Could you check a few things on this model? Use its own coordinates, in mm. A direction names the side the tool comes from. Coordinates: 2 decimals unless noted, no trailing zeros. Loops run counter-clockwise (first coordinate to the right, second up) from the corner with the lowest first, then second, coordinate; pieces in that order, holes last. Notation, with made-up numbers: (89, 54.25) -> (134, 54.25) arc R23 cw to (134, 86.25) -> close; hole circle Ø5 at (-25, 63). An arc over 180 degrees is marked (long way). One line per question, with ' | ' between items.
```python
from build123d import *

# Parameters (mm, degrees)
SKETCH1_R           = 8
BOSS_EXTRUDE1_DEPTH = 67
SKETCH2_R           = 3
BOSS_EXTRUDE2_DEPTH = 2.5
SKETCH3_R           = 3
BOSS_EXTRUDE3_DEPTH = 2.5
SKETCH4_R           = 2
BOSS_EXTRUDE4_DEPTH = 13


with BuildPart() as part:
    # Sketch1 → Boss-Extrude1 (new body)
    with BuildSketch(Plane.XY):
        Circle(SKETCH1_R)
    extrude(amount=BOSS_EXTRUDE1_DEPTH)

    # Sketch2 → Boss-Extrude2 (add)
    with BuildSketch(Plane.XY.offset(67)):
        Circle(SKETCH2_R)
    extrude(amount=BOSS_EXTRUDE2_DEPTH)

    # Sketch3 → Boss-Extrude3 (add)
    with BuildSketch(Plane(origin=(0, 0, 0), x_dir=(-1, 0, 0), z_dir=(0, 0, -1))):
        Circle(SKETCH3_R)
    extrude(amount=BOSS_EXTRUDE3_DEPTH)

    # Sketch4 → Boss-Extrude4 (add)
    with BuildSketch(Plane(origin=(0, 0, -2.5), x_dir=(-1, 0, 0), z_dir=(0, 0, -1))):
        Circle(SKETCH4_R)
    extrude(amount=BOSS_EXTRUDE4_DEPTH)


solid = part.part
```
Q1. Imagine slicing it at D-D on z = -4.5. Write out the boundary of the cut face in (x, y), plus the area to 3 significant figures.
Values follow:
outline: circle Ø4 at (0, 0) | area: 12.6 mm2
Q2. Please list where these lines run through material, in increasing order: L1, parallel to Z at x = 1.5, y = -6.5; L2, parallel to Y at x = -7, z = 1; L3, parallel to Y at x = -5.25, z = 28. Write a range as [from, to].
Values follow:
L1: z = [0, 67] | L2: y = [-3.87, 3.87] | L3: y = [-6.04, 6.04]
Q3. For faces 1 (the face through (0, 0, 69.5)), 2 (the face through (0, -2, -9)), 3 (the face through (3.4, 0.1, 67)), which set-ups out of +Z, -Z, +X, -X, +Y, -Y let a thin tool reach every point of the face, with its end or its side?
Values follow:
face 1: +Z, +X, -X, +Y, -Y | face 2: -Z | face 3: +Z
Q4. Imagine slicing it at C-C on z = 51.5. Write out the boundary of the cut face in (x, y).
Values follow:
outline: circle Ø16 at (0, 0)
Q5. Imagine slicing it at A-A on x = 0. Write out the boundary of the cut face in (y, z), plus the area to 3 significant figures.
Values follow:
outline: (-8, 0) -> (-3, 0) -> (-3, -2.5) -> (-2, -2.5) -> (-2, -15.5) -> (2, -15.5) -> (2, -2.5) -> (3, -2.5) -> (3, 0) -> (8, 0) -> (8, 67) -> (3, 67) -> (3, 69.5) -> (-3, 69.5) -> (-3, 67) -> (-8, 67) -> close | area: 1,150 mm2
Q6. For pin 1 (1 mm diameter, centred on x = -4.5, z = 55, fed in from +Y); pin 2 (3 mm diameter, centred on x = -2, y = 4.5, fed in from -Z); pin 3 (5 mm diameter, centred on x = 4.5, z = 45, fed in from -Y), each with a flat end and sliding along its axis, tell me the tip position at first contact or that it passes through.
Values follow:
pin 1: stops at y = 6.93 | pin 2: stops at z = 0 | pin 3: stops at y = -7.75
